The model under review builds one solid part; all positions refer to its coordinate system, in mm. Coordinates: 2 decimals unless noted, no trailing zeros. Write each loop counter-clockwise with the first axis right and the second up, starting at its lowest first coordinate (ties: lowest second). Pieces come first, ordered by that corner, then holes.
1) For line 1 (X direction, y = -3.8, z = -10); line 2 (X direction, y = -2, z = -25); line 3 (X direction, y = -2.1, z = 16), list the stretches that pass through material, from the lowest coordinate up.
2) Add section D-D, the plane z = -1. State the section outline as (x, y) points, then the cut area to 3 significant figures.
3) Add section C-C, the plane y = -1.6. State the section outline as (x, z) points, then the cut area to 3 significant figures.
4) Add section A-A, the plane x = -11. State the section outline as (y, z) points, then the cut area to 3 significant figures.
5) Add section B-B, the plane z = 32. State the section outline as (x, y) points.
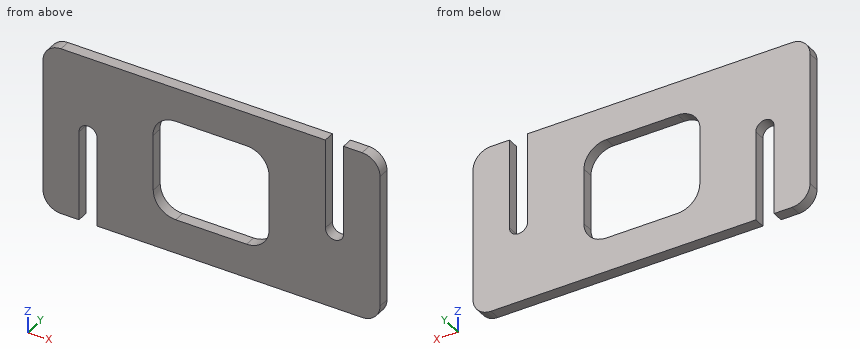
from build123d import *

# Parameters (mm, degrees)
F1_DEPTH = 5
F3_DEPTH = 25
F5_DEPTH = 73
F7_DEPTH = 25


with BuildPart() as f1:
    # F0 (on Front) → F1 (new body)
    with BuildSketch(Plane.XZ):
        with BuildLine():
            ThreePointArc((-66.9997713815, 36.9462131122), (-72.656625631, 34.6030673617), (-74.9997713815, 28.9462131122))
            Line((-74.9997713815, 28.9462131122), (-74.9997713815, -30.0537868878))
            ThreePointArc((-74.9997713815, -30.0537868878), (-72.656625631, -35.7106411373), (-66.9997713815, -38.0537868878))
            Line((-66.9997713815, -38.0537868878), (67.0002286185, -38.0537868878))
            ThreePointArc((67.0002286185, -38.0537868878), (72.657082868, -35.7106411373), (75.0002286185, -30.0537868878))
            Line((75.0002286185, -30.0537868878), (75.0002286185, 28.9462131122))
            ThreePointArc((75.0002286185, 28.9462131122), (72.657082868, 34.6030673617), (67.0002286185, 36.9462131122))
            Line((67.0002286185, 36.9462131122), (-66.9997713815, 36.9462131122))
        make_face()
    extrude(amount=F1_DEPTH)

    # F2 (on face) → F3 (cut)
    with BuildSketch(Plane.XZ.offset(5)):
        with BuildLine():
            Line((-58.9997713815, 1.9462131122), (-58.9997713815, -38.0537868878))
            Line((-58.9997713815, -38.0537868878), (-50.8812127065, -38.0537868878))
            Line((-50.8812127065, -38.0537868878), (-50.8812127065, 1.9462131122))
            ThreePointArc((-50.8812127065, 1.9462131122), (-54.940492044, 6.0054924497), (-58.9997713815, 1.9462131122))
        make_face()
    extrude(amount=-F3_DEPTH, mode=Mode.SUBTRACT)

    # F4 (on face) → F5 (cut)
    with BuildSketch(Plane.XZ.offset(5)):
        with BuildLine():
            Line((58.7657689438, -3.0537868878), (58.7657689438, 36.9462131122))
            Line((58.7657689438, 36.9462131122), (50.6537689438, 36.9462131122))
            Line((50.6537689438, 36.9462131122), (50.6537689438, -3.0537868878))
            ThreePointArc((50.6537689438, -3.0537868878), (54.7097689438, -7.1097868878), (58.7657689438, -3.0537868878))
        make_face()
    extrude(amount=-F5_DEPTH, mode=Mode.SUBTRACT)

    # F6 (on face) → F7 (cut)
    with BuildSketch(Plane.XZ.offset(5)):
        with BuildLine():
            ThreePointArc((25.6149837678, 11.9573603601), (22.6821155465, 19.0212209736), (15.6149899808, 21.9462131122))
            Line((15.6149899808, 21.9462131122), (-16.0960132249, 21.9462131122))
            ThreePointArc((-16.0960132249, 21.9462131122), (-23.1889002898, 18.9953941344), (-26.0958222031, 11.8844037291))
            Line((-26.0958222031, 11.8844037291), (-25.942641223, -12.897926457))
            ThreePointArc((-25.942641223, -12.897926457), (-22.992013267, -19.9290041388), (-15.9428322448, -22.8361170739))
            Line((-15.9428322448, -22.8361170739), (15.6426154759, -22.8361170739))
            ThreePointArc((15.6426154759, -22.8361170739), (22.7176233373, -19.9032426395), (25.6426092628, -12.824969826))
            Line((25.6426092628, -12.824969826), (25.6149837678, 11.9573603601))
        make_face()
    extrude(amount=-F7_DEPTH, mode=Mode.SUBTRACT)


solid = f1.part
Geometry results:
1. line 1: x = -75 to -59, -50.88 to -25.96, 25.64 to 75
1. line 2: x = -75 to -59, -50.88 to 75
1. line 3: x = -75 to -25.24, 24.76 to 50.65, 58.77 to 75
2. outline: (-75, -5) - (-59, -5) - (-59, 0) - (-75, 0) - close; (-50.88, -5) - (-26.02, -5) - (-26.02, 0) - (-50.88, 0) - close; (25.63, -5) - (50.65, -5) - (50.65, 0) - (25.63, 0) - close; (58.77, -5) - (75, -5) - (75, 0) - (58.77, 0) - close
2. area: 411 mm2
3. outline: (-75, -30.05) arc R8 ccw to (-67, -38.05) - (-59, -38.05) - (-59, 1.95) arc R4.06 cw to (-50.88, 1.95) - (-50.88, -38.05) - (67, -38.05) arc R8 ccw to (75, -30.05) - (75, 28.95) arc R8 ccw to (67, 36.95) - (58.77, 36.95) - (58.77, -3.05) arc R4.06 cw to (50.65, -3.05) - (50.65, 36.95) - (-67, 36.95) arc R8 ccw to (-75, 28.95) - close; hole (-26.1, 11.88) - (-25.94, -12.9) arc R10 ccw to (-15.94, -22.84) - (15.64, -22.84) arc R10 ccw to (25.64, -12.82) - (25.61, 11.96) arc R10 ccw to (15.61, 21.95) - (-16.1, 21.95) arc R10 ccw to start
3. area: 8,270 mm2
4. outline: (-5, -38.05) - (0, -38.05) - (0, -22.84) - (-5, -22.84) - close; (-5, 21.95) - (0, 21.95) - (0, 36.95) - (-5, 36.95) - close
4. area: 151 mm2
5. outline: (-74.39, -5) - (50.65, -5) - (50.65, 0) - (-74.39, 0) - close; (58.77, -5) - (74.39, -5) - (74.39, 0) - (58.77, 0) - close
